Check sheet for the modelled part. Datum: model origin and axes. Units: mm. Give positions to 0.01 mm unless a question says otherwise; leave off trailing zeros. Loops run counter-clockwise (first coordinate to the right, second up) from the corner with the lowest first, then second, coordinate; pieces in that order, holes last. Notation, with made-up numbers: (40.25, 47) -> (56.25, 47) arc R20 cw to (56.25, 82) -> close; hole circle Ø11 at (-22, 0.5). An arc over 180 degrees is marked (long way). Answer as CSV lines item,"result". Start each with the question number.
(1) Section check D-D on z = 1. Enter the section's corners in (x, y), plus the area to 3 significant figures.
(2) Material ranges on line 1 (Y direction, x = 46, z = 0.8); line 2 (X direction, y = 10, z = 1.3); line 3 (X direction, y = -0.5, z = 0.6), recorded low to high. Write a range as from..to.
(3) Section check B-B on y = 20. Enter the section's corners in (x, z), plus the area to 3 significant figures.
(4) Section check C-C on x = 46. Enter the section's corners in (y, z).
(5) Section check A-A on y = -20. Enter the section's corners in (x, z).
(6) Gauge pin test, flat ends, axial feed: pin 1 Ø1.6 at (x, z) = (4.5, 1) entering from +Y; pin 2 Ø4.5 at (x, y) = (46, -20) entering from +Z; pin 3 Ø0.5 at (y, z) = (-3, 2.5) entering from +X. Record the tip position at first contact, or that the pin passes through.
from build123d import *

# Parameters (mm, degrees)
EXTRUDE_1_DEPTH     = 3
SKETCH_3_R          = 2
CUT_EXTRUDE_2_DEPTH = 10
FILLET_2_R          = 5
CHAMFER_1_SIZE      = 10
CUT_EXTRUDE_3_DEPTH = 1


with BuildPart() as part:
    # ｽｹｯﾁ1 → ﾎﾞｽ - 押し出し1 (new body)
    with BuildSketch(Plane.XY):
        Polygon((-56, 30), (-56, -30), (56, -30), (56, 30), (36, 30), (36, -10), (-36, -10), (-36, 30), align=None)
    extrude(amount=EXTRUDE_1_DEPTH)

    # ｽｹｯﾁ3 → ｶｯﾄ - 押し出し2 (cut)
    with BuildSketch(Plane.XY.offset(3)):
        with Locations((-46, -20)):
            Circle(SKETCH_3_R)
        with Locations((46, -20)):
            Circle(SKETCH_3_R)
        with Locations((46, 0)):
            Circle(SKETCH_3_R)
        with Locations((-46, 0)):
            Circle(SKETCH_3_R)
        with Locations((-46, 20)):
            Circle(SKETCH_3_R)
        with Locations((46, 20)):
            Circle(SKETCH_3_R)
    extrude(amount=-CUT_EXTRUDE_2_DEPTH, mode=Mode.SUBTRACT)

    # ﾌｨﾚｯﾄ2
    fillet_2_edges = [part.edges().sort_by_distance(p)[0] for p in [
        (36, 30, 1.5),
        (56, 30, 1.5),
        (56, -30, 1.5),
        (-56, -30, 1.5),
        (-56, 30, 1.5),
        (-36, 30, 1.5),
    ]]
    fillet(fillet_2_edges, radius=FILLET_2_R)

    # 面取り1
    chamfer_1_edges = [part.edges().sort_by_distance(p)[0] for p in [
        (36, -10, 1.5),
        (-36, -10, 1.5),
    ]]
    chamfer(chamfer_1_edges, length=CHAMFER_1_SIZE)

    # ｽｹｯﾁ4 → ｶｯﾄ - 押し出し3 (cut)
    with BuildSketch(Plane.XY.offset(3)):
        with BuildLine():
            Line((-36, 0), (-36, -10))
            Line((-36, -10), (-26, -10))
            Line((-26, -10), (26, -10))
            Line((26, -10), (36, -10))
            Line((36, -10), (36, 0))
            Line((36, 0), (36, 25))
            ThreePointArc((36, 25), (37.464466094, 28.535533906), (41, 30))
            Line((41, 30), (51, 30))
            ThreePointArc((51, 30), (54.535533906, 28.535533906), (56, 25))
            Line((56, 25), (56, -25))
            ThreePointArc((56, -25), (54.535533906, -28.535533906), (51, -30))
            Line((51, -30), (-51, -30))
            ThreePointArc((-51, -30), (-54.535533906, -28.535533906), (-56, -25))
            Line((-56, -25), (-56, 25))
            ThreePointArc((-56, 25), (-54.535533906, 28.535533906), (-51, 30))
            Line((-51, 30), (-41, 30))
            ThreePointArc((-41, 30), (-37.464466094, 28.535533906), (-36, 25))
            Line((-36, 25), (-36, 0))
        make_face()
    extrude(amount=-CUT_EXTRUDE_3_DEPTH, mode=Mode.SUBTRACT)


solid = part.part
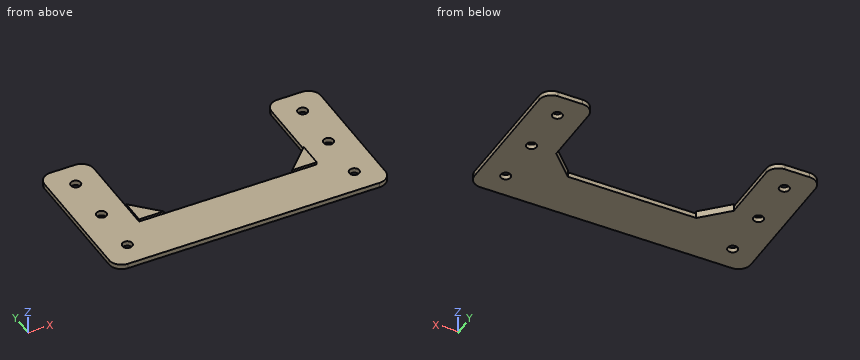
Working result:
1,outline,"(-56, -25) arc R5 ccw to (-51, -30) -> (51, -30) arc R5 ccw to (56, -25) -> (56, 25) arc R5 ccw to (51, 30) -> (41, 30) arc R5 ccw to (36, 25) -> (36, 0) -> (26, -10) -> (-26, -10) -> (-36, 0) -> (-36, 25) arc R5 ccw to (-41, 30) -> (-51, 30) arc R5 ccw to (-56, 25) -> close; hole circle Ø4 at (-46, -20); hole circle Ø4 at (-46, 0); hole circle Ø4 at (-46, 20); hole circle Ø4 at (46, -20); hole circle Ø4 at (46, 0); hole circle Ø4 at (46, 20)"
1,area,"3,830 mm^2"
2,line 1,"y = -30..-22, -18..-2, 2..18, 22..30"
2,line 2,"x = -56..-36, 36..56"
2,line 3,"x = -56..-47.94, -44.06..-35.5, 35.5..44.06, 47.94..56"
3,outline,"(-56, 0) -> (-48, 0) -> (-48, 2) -> (-56, 2) -> close; (-44, 0) -> (-36, 0) -> (-36, 2) -> (-44, 2) -> close; (36, 0) -> (44, 0) -> (44, 2) -> (36, 2) -> close; (48, 0) -> (56, 0) -> (56, 2) -> (48, 2) -> close"
3,area,"64.0 mm^2"
4,outline,"(-30, 0) -> (-22, 0) -> (-22, 2) -> (-30, 2) -> close; (-18, 0) -> (-2, 0) -> (-2, 2) -> (-18, 2) -> close; (2, 0) -> (18, 0) -> (18, 2) -> (2, 2) -> close; (22, 0) -> (30, 0) -> (30, 2) -> (22, 2) -> close"
5,outline,"(-56, 0) -> (-48, 0) -> (-48, 2) -> (-56, 2) -> close; (-44, 0) -> (44, 0) -> (44, 2) -> (-44, 2) -> close; (48, 0) -> (56, 0) -> (56, 2) -> (48, 2) -> close"
6,pin 1,"stops at y = -10"
6,pin 2,"stops at z = 2"
6,pin 3,"stops at x = 36"
